Verification items for the finished model (mm, model axes). A direction names the side the tool comes from. Round coordinates to 2 decimals unless told otherwise and drop trailing zeros. Write each loop counter-clockwise with the first axis right and the second up, starting at its lowest first coordinate (ties: lowest second). Pieces come first, ordered by that corner, then holes. Notation, with made-up numbers: M 24,-16.5 L 80,-16.5 A15 ccw 80,-7.5 Z; hole C 21,-39.5 d5. An arc over 180 degrees is marked long. Write each question's results on one line, items separated by ' | '.
from build123d import *

# Parameters (mm, degrees)
F1_DEPTH = 3
F2_DEPTH = 12
F3_DEPTH = 50
F5_DEPTH = 3


with BuildPart() as f1:
    # F0 (on Top) → F1 (new body)
    with BuildSketch(Plane.XY):
        with BuildLine():
            Line((15.75, -23.5), (15.75, 0))
            ThreePointArc((15.75, 0), (0, 15.75), (-15.75, 0))
            Line((-15.75, 0), (-15.75, -23.5))
            ThreePointArc((-15.75, -23.5), (0, -39.25), (15.75, -23.5))
        make_face()
        with BuildLine():
            ThreePointArc((-12.75, 0), (0, 12.75), (12.75, 0))
            Line((12.75, 0), (12.75, -23.5))
            ThreePointArc((12.75, -23.5), (0, -36.25), (-12.75, -23.5))
            Line((-12.75, -23.5), (-12.75, 0))
        make_face(mode=Mode.SUBTRACT)
        with BuildLine():
            ThreePointArc((-12.75, 0), (0, -12.75), (12.75, 0))
            ThreePointArc((12.75, 0), (0, 12.75), (-12.75, 0))
        make_face()
        with BuildLine():
            Line((12.75, -23.5), (12.75, 0))
            ThreePointArc((12.75, 0), (0, -12.75), (-12.75, 0))
            Line((-12.75, 0), (-12.75, -23.5))
            ThreePointArc((-12.75, -23.5), (0, -36.25), (12.75, -23.5))
        make_face()
    extrude(amount=F1_DEPTH)

    # F0 (on Top) → F2 (join)
    with BuildSketch(Plane.XY):
        with BuildLine():
            Line((12.75, -23.5), (12.75, 0))
            ThreePointArc((12.75, 0), (0, -12.75), (-12.75, 0))
            Line((-12.75, 0), (-12.75, -23.5))
            ThreePointArc((-12.75, -23.5), (0, -36.25), (12.75, -23.5))
        make_face()
    extrude(amount=F2_DEPTH)

    # F0 (on Top) → F3 (join)
    with BuildSketch(Plane.XY):
        with BuildLine():
            Line((15.75, -23.5), (15.75, 0))
            ThreePointArc((15.75, 0), (0, 15.75), (-15.75, 0))
            Line((-15.75, 0), (-15.75, -23.5))
            ThreePointArc((-15.75, -23.5), (0, -39.25), (15.75, -23.5))
        make_face()
        with BuildLine():
            ThreePointArc((-12.75, 0), (0, 12.75), (12.75, 0))
            Line((12.75, 0), (12.75, -23.5))
            ThreePointArc((12.75, -23.5), (0, -36.25), (-12.75, -23.5))
            Line((-12.75, -23.5), (-12.75, 0))
        make_face(mode=Mode.SUBTRACT)
    extrude(amount=F3_DEPTH)

    # F4 (on face) → F5 (join)
    with BuildSketch(Plane.XY.offset(50)):
        with BuildLine():
            ThreePointArc((14.25, 0), (0, 14.25), (-14.25, 0))
            Line((-14.25, 0), (-14.25, -23.5))
            ThreePointArc((-14.25, -23.5), (0, -37.75), (14.25, -23.5))
            Line((14.25, -23.5), (14.25, 0))
        make_face()
        with BuildLine():
            ThreePointArc((-12.75, 0), (0, 12.75), (12.75, 0))
            Line((12.75, 0), (12.75, -23.5))
            ThreePointArc((12.75, -23.5), (0, -36.25), (-12.75, -23.5))
            Line((-12.75, -23.5), (-12.75, 0))
        make_face(mode=Mode.SUBTRACT)
    extrude(amount=F5_DEPTH)


solid = f1.part
1) Sectioned sample at A-A, the plane z = 37.5. Record the cut outline in (x, y), and give its area (3 significant figures).
Calculated:
outline: M -15.75,-23.5 A15.75 ccw 15.75,-23.5 L 15.75,0 A15.75 ccw -15.75,0 Z; hole M -12.75,-23.5 A12.75 ccw 12.75,-23.5 L 12.75,0 A12.75 ccw -12.75,0 Z | area: 410 mm²
2) Depth check by flat-ended pin: P1, Ø8, axis at y = 0.5, z = 11, coming from the +X side; P2, Ø4, axis at x = -7, z = 28.5, coming from the -Y side; P3, Ø10, axis at x = -0.5, y = -11.5, coming from the +Z side; P4, Ø3, axis at x = 11, z = 8, coming from the +Y side. Enter the tip coordinate at first touch or a pass-through.
Calculated:
P1: stops at x = 15.75 | P2: stops at y = -38.44 | P3: stops at z = 12 | P4: stops at y = 12.56
3) Material ranges on line 1 (X direction, y = -18.5, z = 31); line 2 (Y direction, x = 0, z = 15); line 3 (Y direction, x = 0, z = 9), recorded low to high. Write a range as [from, to].
Calculated:
line 1: x = [-15.75, -12.75], [12.75, 15.75] | line 2: y = [-39.25, -36.25], [12.75, 15.75] | line 3: y = [-39.25, -12.75], [12.75, 15.75]
4) Draft check along X on faces 4 (the flat face through (0, 0, 3)), 5 (the flat face through (-14, -12, 53)), 6 (the cylindrical face through (1.66, 12.64, 22.09)), 7 (the cylindrical face through (0.346, 15.746, 24.65)). Enter one of: pulls with the +X half, pulls with the -X half, needs draft (parallel to the pull), parting line crosses it, or undercut.
Calculated:
face 4: undercut | face 5: needs draft | face 6: undercut | face 7: parting line crosses it
5) Sectioned sample at D-D, the plane y = -32. Record the cut outline in (x, z), and give its area (3 significant figures).
Calculated:
outline: M -13.26,0 L 13.26,0 L 13.26,50 L 11.44,50 L 11.44,53 L 9.5,53 L 9.5,12 L -9.5,12 L -9.5,53 L -11.44,53 L -11.44,50 L -13.26,50 Z | area: 615 mm²
6) Access from +Z, -Z, +X, -X, +Y, -Y to the whole of each face (thin tool, end or side, straight path). Record for faces 1 (the flat face through (12.75, -12, 32)), 2 (the flat face through (-14.25, -12, 51)), 3 (the flat face through (14.25, -12, 51)).
Calculated:
face 1: +Z | face 2: +Z, -X, +Y, -Y | face 3: +Z, +X, +Y, -Y
7) Sectioned sample at B-B, the plane x = 0. Record the cut outline in (y, z).
Calculated:
outline: M -39.25,0 L 15.75,0 L 15.75,50 L 14.25,50 L 14.25,53 L 12.75,53 L 12.75,3 L -12.75,3 L -12.75,12 L -36.25,12 L -36.25,53 L -37.75,53 L -37.75,50 L -39.25,50 Z
8) Sectioned sample at C-C, the plane y = -18. Record the cut outline in (x, z), and give its area (3 significant figures).
Calculated:
outline: M -15.75,0 L 15.75,0 L 15.75,50 L 14.25,50 L 14.25,53 L 12.75,53 L 12.75,12 L -12.75,12 L -12.75,53 L -14.25,53 L -14.25,50 L -15.75,50 Z | area: 615 mm²
